Autodesk Inventor part; units mm, degrees
ref_plane "YZ Plane" through (0, 0, 0) normal (1, 0, 0) x (0, 1, 0)
ref_plane "XZ Plane" through (0, 0, 0) normal (0, 1, 0) x (-1, 0, 0)
ref_plane "XY Plane" through (0, 0, 0) normal (0, 0, 1) x (1, 0, 0)
sketch "Sketch6" plane through (0, 0, 0) normal (0, 0, 1) x (1, 0, 0)
  line L0 (19.5, -12.4999) -> (-19.5, -12.4999)
  line L1 (-19.5, -12.4999) -> (-19.5, 12.4999)
  line L2 (19.5, 12.4999) -> (19.5, -12.4999)
  line L3 (19.5, -12.4999) -> (-19.5, 12.4999) construction
  line L4 (-19.5, -12.4999) -> (19.5, 12.4999) construction
  line L5 (5.4997, 12.4999) -> (5.4997, 17.5003)
  line L6 (5.4997, 17.5003) -> (19.5, 17.5003)
  line L7 (19.5, 17.5003) -> (19.5, 12.4999)
  line L8 (1.9998, 6.5001) -> (0.0002, 6.5001)
  line L9 (0.0002, 6.5001) -> (0.0002, 12.4999)
  line L10 (1.9998, 12.4999) -> (1.9998, 6.5001)
  line L11 (1.9998, 6.5001) -> (0.0002, 12.4999) construction
  line L12 (0.0002, 6.5001) -> (1.9998, 12.4999) construction
  line L13 (-19.5, 12.4999) -> (0.0002, 12.4999)
  line L14 (1.9998, 12.4999) -> (5.4997, 12.4999)
extrude "Extrusion5" add sketch "Sketch6" along normal blind 1.6
fillet "Fillet5" radius 2 4 edges at (19.5, 17.5003, 0.8) (-19.5, 12.4999, 0.8) (-19.5, -12.4999, 0.8) (19.5, -12.4999, 0.8)
properties part number "pcb_balun_bottom"
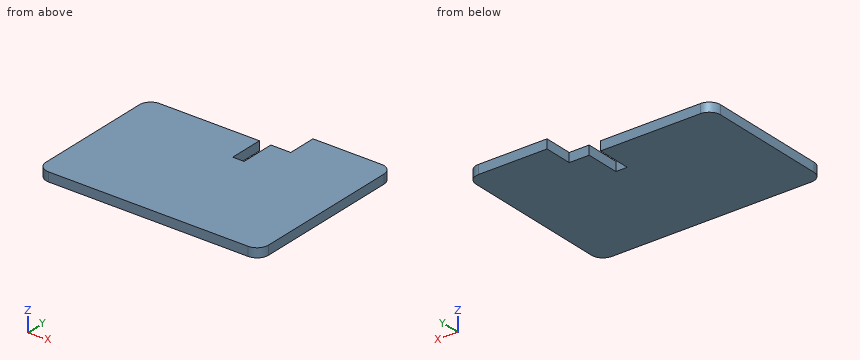
Can you work these out from the model? Positions are in its coordinate system, mm. Round coordinates to 2 decimals unless told otherwise and drop trailing zeros. Write each loop counter-clockwise with the first axis right and the second up, starting at its lowest first coordinate (ties: lowest second). Pieces come first, ordered by that corner, then holes. Notation, with made-up numbers: (-33, -21.75) -> (-14, -21.75) arc R8 cw to (-14, -8.75) -> close; hole circle Ø5 at (86, -7.5). An arc over 180 degrees is marked (long way). One line per question, with ' | ' between items. Start each with the question number.
1) Suppose I cut it at A-A on y = 9.5. Write out the boundary of the cut face in (x, z).
2) Suppose I cut it at C-C on x = 1.5. Write out the boundary of the cut face in (y, z), then the cut area to 3 significant figures.
3) I'm going to push flat-ended pins straight in: P1, Ø0.5, axis at x = 1, z = 0.5, coming from the +Y side; P2, Ø3, axis at x = -4.5, y = -1, coming from the -Z side; P3, Ø0.5, axis at x = -13, z = 1, coming from the +Y side; P4, Ø0.8, axis at y = 14, z = 0.5, coming from the -X side. Where does each tip first touch, or does it pass through?
4) Suppose I cut it at D-D on y = 14. Write out the boundary of the cut face in (x, z).
5) Suppose I cut it at B-B on z = 1.3. Write out the boundary of the cut face in (x, y).
6) I need wall thicknesses on line 1 (Y direction, x = -10.5, z = 0.4); line 2 (X direction, y = 9, z = 1.4); line 3 (X direction, y = 15.5, z = 0.3). Which ranges of each line are inside material? Lowest first, please. Write a range as [from, to].
Return value:
1) outline: (-19.5, 0) -> (0, 0) -> (0, 1.6) -> (-19.5, 1.6) -> close; (2, 0) -> (19.5, 0) -> (19.5, 1.6) -> (2, 1.6) -> close
2) outline: (-12.5, 0) -> (6.5, 0) -> (6.5, 1.6) -> (-12.5, 1.6) -> close | area: 30.4 mm2
3) P1: stops at y = 6.5 | P2: stops at z = 0 | P3: stops at y = 12.5 | P4: stops at x = 5.5
4) outline: (5.5, 0) -> (19.5, 0) -> (19.5, 1.6) -> (5.5, 1.6) -> close
5) outline: (-19.5, -10.5) arc R2 ccw to (-17.5, -12.5) -> (17.5, -12.5) arc R2 ccw to (19.5, -10.5) -> (19.5, 15.5) arc R2 ccw to (17.5, 17.5) -> (5.5, 17.5) -> (5.5, 12.5) -> (2, 12.5) -> (2, 6.5) -> (0, 6.5) -> (0, 12.5) -> (-17.5, 12.5) arc R2 ccw to (-19.5, 10.5) -> close
6) line 1: y = [-12.5, 12.5] | line 2: x = [-19.5, 0], [2, 19.5] | line 3: x = [5.5, 19.5]
